Verification items for the finished model (mm, model axes). A direction names the side the tool comes from. Coordinates: 2 decimals unless noted, no trailing zeros. Order: outer loops, then holes, each group sorted by start corner. A loop starts at its lowest first (then second) coordinate and runs counter-clockwise, first axis right, second up. Notation, with made-up numbers: (-8.75, 35) -> (20.25, 35) arc R21 cw to (20.25, 43) -> close; hole circle Ø5 at (77.5, 10). An arc over 180 degrees is marked (long way). Write item = value, one per line. Start each with the question number.
1. Cross-section at D-D on y = -23.25. Record the cut outline in (x, z), plus the area to 3 significant figures.
2. Cross-section at C-C on y = -15.75. Record the cut outline in (x, z), plus the area to 3 significant figures.
3. Cross-section at B-B on x = 54. Record the cut outline in (y, z).
4. Go/stop test with a flat-tipped pin: P1, Ø4, axis at y = -16, z = 29, coming from the +X side. Record where the tip stops, or that it passes through.
5. Thickness scan on line 1 along Z through (x, y) = (56, -17.25); line 2 along Y through (x, z) = (52, -3); line 3 along Y through (x, z) = (44, 33.5). Record the ranges inside material, lowest first. Write a range as from..to.
6. Release check for a two-part mould opening along Z. For faces 1 (the flat face through (56, -15, -6.279)), 2 (the flat face through (-1, 0, 0)), 3 (the cylindrical face through (0.889, -1.528, 36.651)) record: +Z half, -Z half, draft (parallel to the pull), parting line (faces both ways), or undercut.
7. Cross-section at A-A on z = 4. Record the cut outline in (x, y), plus the area to 3 significant figures.
8. Set-up check for faces 4 (the flat face through (56, -18.789, 1)), 5 (the flat face through (-1, -25.4, 0)): record each of +Z, -Z, +X, -X, +Y, -Y from which the full face is reachable in a straight line by a thin tool's end or side.
from build123d import *

# Parameters (mm, degrees)
F0_W     = 127
F0_H     = 76.2
F1_DEPTH = 25.4
F2_R     = 5.08
F3_W     = 7
F3_H     = 13.8
F4_DEPTH = 15
F5_W     = 7
F5_H     = 13.8
F6_DEPTH = 15


with BuildPart() as f1:
    # F0 (on Front) → F1 (new body)
    with BuildSketch(Plane.XZ):
        Rectangle(F0_W, F0_H)
    extrude(amount=F1_DEPTH)

    # F2
    f2_edges = [f1.edges().sort_by_distance(p)[0] for p in [
        (0, -25.4, 38.1),
        (0, 0, 38.1),
        (0, -25.4, -38.1),
        (0, 0, -38.1),
    ]]
    fillet(f2_edges, radius=F2_R)

    # F3 (on face) → F4 (cut)
    with BuildSketch(Plane.YZ.offset(63.5)):
        with Locations((-15.288545, 26.12)):
            Rectangle(F3_W, F3_H)
    extrude(amount=-F4_DEPTH, mode=Mode.SUBTRACT)

    # F5 (on face) → F6 (cut)
    with BuildSketch(Plane.YZ.offset(63.5)):
        with Locations((-15.288545, 0.620681)):
            Rectangle(F5_W, F5_H)
    extrude(amount=-F6_DEPTH, mode=Mode.SUBTRACT)


solid = f1.part
Worked out:
q1.outline = (-63.5, -37.17) -> (63.5, -37.17) -> (63.5, 37.17) -> (-63.5, 37.17) -> close
q1.area = 9,440 mm²
q2.outline = (-63.5, -38.1) -> (63.5, -38.1) -> (63.5, -6.28) -> (48.5, -6.28) -> (48.5, 7.52) -> (63.5, 7.52) -> (63.5, 19.22) -> (48.5, 19.22) -> (48.5, 33.02) -> (63.5, 33.02) -> (63.5, 38.1) -> (-63.5, 38.1) -> close
q2.area = 9,260 mm²
q3.outline = (-25.4, -33.02) arc R5.08 ccw to (-20.32, -38.1) -> (-5.08, -38.1) arc R5.08 ccw to (0, -33.02) -> (0, 33.02) arc R5.08 ccw to (-5.08, 38.1) -> (-20.32, 38.1) arc R5.08 ccw to (-25.4, 33.02) -> close; hole (-18.79, -6.28) -> (-11.79, -6.28) -> (-11.79, 7.52) -> (-18.79, 7.52) -> close; hole (-18.79, 19.22) -> (-11.79, 19.22) -> (-11.79, 33.02) -> (-18.79, 33.02) -> close
q4.P1 = 48.5
q5.line_1 = -38.1..-6.28, 7.52..19.22, 33.02..38.1
q5.line_2 = -25.4..-18.79, -11.79..0
q5.line_3 = -25.38..-0.02
q6.face_1 = undercut
q6.face_2 = draft
q6.face_3 = +Z half
q7.outline = (-63.5, -25.4) -> (63.5, -25.4) -> (63.5, -18.79) -> (48.5, -18.79) -> (48.5, -11.79) -> (63.5, -11.79) -> (63.5, 0) -> (-63.5, 0) -> close
q7.area = 3,120 mm²
q8.face_4 = +X
q8.face_5 = +Z, -Z, +X, -X, -Y
